```python
from build123d import *

# Parameters (mm, degrees)
BOSS_EXTRUDE1_DEPTH                  = 55
CUT_EXTRUDE2_DEPTH                   = 146
F_25_0_25_DIAMETER_HOLE3_D           = 25
F_25_0_25_DIAMETER_HOLE3_CSINK_D     = 25.05
F_25_0_25_DIAMETER_HOLE3_CSINK_ANGLE = 90
F_25_0_25_DIAMETER_HOLE4_D           = 25
F_25_0_25_DIAMETER_HOLE4_CSINK_D     = 25.05
F_25_0_25_DIAMETER_HOLE4_CSINK_ANGLE = 90


with BuildPart() as part:
    # Sketch1 → Boss-Extrude1 (new body)
    with BuildSketch(Plane(origin=(0, 0, 0), x_dir=(1, 0, 0), z_dir=(0, 1, 0))):
        Polygon((0, 0), (90, 0), (90, 30), (120, 30), (120, 60), (102.487310381, 60), (0, 60), align=None)
    extrude(amount=BOSS_EXTRUDE1_DEPTH)

    # Sketch4 → Cut-Extrude2 (cut, through all)
    with BuildSketch(Plane.XY):
        Polygon((60, 55), (120, 0), (120, 55), align=None)
    extrude(amount=-CUT_EXTRUDE2_DEPTH, mode=Mode.SUBTRACT)

    # Ø25.0 (25) Diameter Hole3 (through all)
    with Locations(Plane(origin=(30, 25, 0), x_dir=(1, 0, 0), z_dir=(0, 0, 1))):
        with Locations((0, 0)):
            CounterSinkHole(F_25_0_25_DIAMETER_HOLE3_D / 2, F_25_0_25_DIAMETER_HOLE3_CSINK_D / 2, counter_sink_angle=F_25_0_25_DIAMETER_HOLE3_CSINK_ANGLE)

    # Ø25.0 (25) Diameter Hole4 (through all)
    with Locations(Plane(origin=(30, 55, -30), x_dir=(0, 0, 1), z_dir=(0, 1, 0))):
        with Locations((0, 0)):
            CounterSinkHole(F_25_0_25_DIAMETER_HOLE4_D / 2, F_25_0_25_DIAMETER_HOLE4_CSINK_D / 2, counter_sink_angle=F_25_0_25_DIAMETER_HOLE4_CSINK_ANGLE)


solid = part.part
```
The listing builds one solid part. Answer for the finished solid, in the listing's coordinates (mm). A direction names the side the tool comes from. Round coordinates to 2 decimals unless told otherwise and drop trailing zeros. Loops run counter-clockwise (first coordinate to the right, second up) from the corner with the lowest first, then second, coordinate; pieces in that order, holes last. Notation, with made-up numbers: (-1.5, 43.25) - (57.5, 43.25) arc R24 cw to (57.5, 59.25) - close; hole circle Ø3 at (-12.75, 1). An arc over 180 degrees is marked (long way). Return JSON: item names as keys, results as strings. Group by question number.
1. The part is cut by section A-A on x = 30. Determine the outline of the cut face in (y, z) (3 decimals).
2. The mould has two halves that part along X. Classify faces 1 (the flat face through (44, 27, 0)), 2 (the cylindrical face through (40.54, 9.55, -36.72)), 3 (the flat face through (82.91, 34, -36.25)): pulls with the +X half, pulls with the -X half, needs draft (parallel to the pull), parting line crosses it, or undercut.
3. This flat-tipped pin is pushed along its axis until it touches: P1, Ø10, axis at x = 82.5, z = -42.5, coming from the +Y side. Where does it stop, or does it pass through?
4. The part is cut by section D-D on x = 80. Determine the outline of the cut face in (y, z).
5. The part is cut by section B-B on z = -54.5. Determine the outline of the cut face in (x, y).
6. Consider probe 1 along X at (y, z) = (25, -9); probe 2 along Y at (x, z) = (30, -7); probe 3 along Z at (x, y) = (30, 42.25). Determine where each line is inside the solid, lowest interval first.
7. Which of the six approach directions +Z, -Z, +X, -X, +Y, -Y give full straight-line access (tool end or side, diameter ignored) to faces 4 (the cylindrical face through (42.488, 25.55, -48.543)), 5 (the flat face through (101, 11, -30))?
8. The part is cut by section C-C on y = 49. Determine the outline of the cut face in (x, z), then the cut area to 3 significant figures.
Resolved:
{
 "1": {"outline": "(0, -60) - (12.5, -60) - (12.5, -42.5) - (0, -42.5) - close; (0, -17.5) - (12.5, -17.5) - (12.5, -0.025) - (12.475, 0) - (0, 0) - close; (37.5, -60) - (55, -60) - (55, -42.525) - (54.975, -42.5) - (37.5, -42.5) - close; (37.5, -17.5) - (54.975, -17.5) - (55, -17.475) - (55, 0) - (37.525, 0) - (37.5, -0.025) - close"},
 "2": {"face 1": "needs draft", "face 2": "undercut", "face 3": "pulls with the +X half"},
 "3": {"P1": "stops at y = 38.96"},
 "4": {"outline": "(0, -60) - (36.67, -60) - (36.67, 0) - (0, 0) - close"},
 "5": {"outline": "(0, 0) - (120, 0) - (60, 55) - (0, 55) - close; hole circle Ø25 at (30, 25)"},
 "6": {"probe 1": "x = 0 to 17.5, 42.5 to 90", "probe 2": "y = 0 to 12.5, 37.5 to 55", "probe 3": "z = -60 to -42.5, -17.5 to 0"},
 "7": {"face 4": "+Z, -Z", "face 5": "+Z, +X, +Y, -Y"},
 "8": {"outline": "(0, -60) - (66.55, -60) - (66.55, 0) - (0, 0) - close; hole circle Ø25 at (30, -30)", "area": "3,500 mm²"}
}
